```python
from build123d import *

# Parameters (mm, degrees)
ESQUISSE1_R             = 37
ESQUISSE1_R_2           = 1.5
ESQUISSE1_W             = 25
ESQUISSE1_H             = 3
BOSS_EXTRU_1_DEPTH      = 2
BOSS_EXTRU_2_DEPTH      = 15
ESQUISSE3_W             = 1.5
ESQUISSE3_H             = 28.4
ESQUISSE3_W_2           = 1.2
BOSS_EXTRU_3_DEPTH      = 2
ESQUISSE5_W             = 1.5
ESQUISSE5_H             = 24.4
ESQUISSE5_W_2           = 1.2
BOSS_EXTRU_4_DEPTH      = 2
ESQUISSE10_R            = 2
ENL_V_MAT_EXTRU_3_DEPTH = 49
ENL_V_START             = -2
ESQUISSE11_R            = 37
ENL_V_MAT_EXTRU_4_DEPTH = 2
SKETCH4_R               = 3.5
CUT_EXTRUDE2_DEPTH      = 3


with BuildPart() as part:
    # Esquisse1 → Boss.-Extru.1 (new body)
    with BuildSketch(Plane.XY):
        Circle(ESQUISSE1_R)
        with Locations((0, 30)):
            Circle(ESQUISSE1_R_2, mode=Mode.SUBTRACT)
        with Locations((-25.416453209, -15.9375)):
            Circle(ESQUISSE1_R_2, mode=Mode.SUBTRACT)
        with Locations((0, -27)):
            Circle(ESQUISSE1_R_2, mode=Mode.SUBTRACT)
        with Locations((25.416453209, -15.9375)):
            Circle(ESQUISSE1_R_2, mode=Mode.SUBTRACT)
        with Locations((0, -15.5)):
            Rectangle(ESQUISSE1_W, ESQUISSE1_H, mode=Mode.SUBTRACT)
    extrude(amount=BOSS_EXTRU_1_DEPTH)

    # Esquisse2 → Boss.-Extru.2 (add)
    with BuildSketch(Plane(origin=(0, 0, 0), x_dir=(-1, 0, 0), z_dir=(0, 0, -1))):
        Polygon((-22.55, 14.9), (-12.55, 14.9), (-12.55, -9.5), (12.55, -9.5), (12.55, 14.9), (22.55, 14.9), (22.55, -13.5), (-22.55, -13.5), align=None)
    extrude(amount=BOSS_EXTRU_2_DEPTH)

    # Esquisse3 → Boss.-Extru.3 (add)
    with BuildSketch(Plane(origin=(-12.55, 0, 0), x_dir=(0, 0, -1), z_dir=(1, 0, 0))):
        with Locations((9.375, 0.7)):
            Rectangle(ESQUISSE3_W, ESQUISSE3_H)
        with Locations((6.825, 0.7)):
            Rectangle(ESQUISSE3_W_2, ESQUISSE3_H)
    extrude(amount=BOSS_EXTRU_3_DEPTH)

    # Esquisse5 → Boss.-Extru.4 (add)
    with BuildSketch(Plane.ZY.offset(-12.55)):
        with Locations((-9.375, 2.7)):
            Rectangle(ESQUISSE5_W, ESQUISSE5_H)
        with Locations((-6.825, 2.7)):
            Rectangle(ESQUISSE5_W_2, ESQUISSE5_H)
    extrude(amount=BOSS_EXTRU_4_DEPTH)

    # Esquisse10 → Enlèv. mat.-Extru.3 (cut)
    with BuildSketch(Plane.XY.offset(2)):
        with Locations((-17.55, 8.9)):
            Circle(ESQUISSE10_R)
        with Locations((-17.55, -8.5)):
            Circle(ESQUISSE10_R)
        with Locations((17.55, -8.5)):
            Circle(ESQUISSE10_R)
        with Locations((17.55, 8.9)):
            Circle(ESQUISSE10_R)
    extrude(amount=-ENL_V_MAT_EXTRU_3_DEPTH, mode=Mode.SUBTRACT)

    # Esquisse11 → Enlèv. mat.-Extru.4 (cut)
    with BuildSketch(Plane.XY.offset(2).offset(ENL_V_START)):
        Circle(ESQUISSE11_R)
    extrude(amount=ENL_V_MAT_EXTRU_4_DEPTH, mode=Mode.SUBTRACT)

    # Sketch4 → Cut-Extrude2 (cut)
    with BuildSketch(Plane(origin=(0, 0, -15), x_dir=(-1, 0, 0), z_dir=(0, 0, -1))):
        with Locations((-17.55, -8.5)):
            Circle(SKETCH4_R)
        with Locations((-17.55, 8.9)):
            Circle(SKETCH4_R)
        with Locations((17.55, 8.9)):
            Circle(SKETCH4_R)
        with Locations((17.55, -8.5)):
            Circle(SKETCH4_R)
    extrude(amount=-CUT_EXTRUDE2_DEPTH, mode=Mode.SUBTRACT)


solid = part.part
```
Could you check a few things on this model? Use its own coordinates, in mm. A direction names the side the tool comes from. Give positions to 0.01 mm unless a question says otherwise; leave off trailing zeros. Order: outer loops, then holes, each group sorted by start corner. A loop starts at its lowest first (then second) coordinate and runs counter-clockwise, first axis right, second up.
Q1. Suppose I cut it at B-B, the plane y = 13. Write out the boundary of the cut face in (x, z) (3 decimals), and give its area (3 significant figures).
Q2. If I drill on line 1 along Y through (x, z) = (-17.55, -2.75); line 2 along Y through (x, z) = (17.55, -13.6); line 3 along X through (y, z) = (-2, -11.5), over which ranges is the centre line in solid material (lowest first)?
Q3. Suppose I cut it at D-D, the plane x = -8.5. Write out the boundary of the cut face in (y, z).
Q4. For faces 1 (the flat face through (10.55, 3, -9)), 2 (the flat face through (-12, 3, -10.125)), 3 (the flat face through (12, 3, -8.625)), 4 (the flat face through (12.55, 3, -3)), 5 (the cylindrical face through (-19.165, -11.605, -13.521)), which set-ups out of +Z, -Z, +X, -X, +Y, -Y let a thin tool reach every point of the face, with its end or its side?
Q5. I'm going to push flat-ended pins straight in: P1, Ø5.5, axis at x = -17.55, y = 8.9, coming from the +Z side; P2, Ø3.5, axis at x = -19, y = -8.5, coming from the -Z side; P3, Ø0.6, axis at x = 11.5, y = 7.5, coming from the +Z side (3 decimals); P4, Ø1.6, axis at x = -11.5, y = 4.5, coming from the -Z side (3 decimals). Where does each tip first touch, or does it pass through?
Q6. We'd pull the mould along X, two halves only. Please class faces 6 (the flat face through (12.55, 3, -13)), 7 (the flat face through (-18, 14.9, -7)): +X half, -X half, draft (parallel to the pull), parting line (faces both ways), or undercut.
Q7. Suppose I cut it at A-A, the plane x = 17.55. Write out the boundary of the cut face in (y, z).
Q8. Suppose I cut it at C-C, the plane z = -4. Write out the boundary of the cut face in (x, y), and give its area (3 significant figures).
Solution:
1. outline: (-22.55, -15) - (-12.55, -15) - (-12.55, -10.125) - (-10.55, -10.125) - (-10.55, -8.625) - (-12.55, -8.625) - (-12.55, -7.425) - (-10.55, -7.425) - (-10.55, -6.225) - (-12.55, -6.225) - (-12.55, 0) - (-22.55, 0) - close; (10.55, -10.125) - (12.55, -10.125) - (12.55, -15) - (22.55, -15) - (22.55, 0) - (12.55, 0) - (12.55, -6.225) - (10.55, -6.225) - (10.55, -7.425) - (12.55, -7.425) - (12.55, -8.625) - (10.55, -8.625) - close
1. area: 311 mm2
2. line 1: y = -13.5 to -10.5, -6.5 to 6.9, 10.9 to 14.9
2. line 2: y = -13.5 to -12, -5 to 5.4, 12.4 to 14.9
2. line 3: x = -22.55 to -12.55, 12.55 to 22.55
3. outline: (-13.5, -15) - (-9.5, -15) - (-9.5, 0) - (-13.5, 0) - close
4. face 1: +Z, -Z, +Y
4. face 2: -Z, +Y
4. face 3: +Y
4. face 4: +Z, +Y
4. face 5: -Z
5. P1: stops at z = 0
5. P2: stops at z = -12
5. P3: stops at z = -6.225
5. P4: stops at z = -10.125
6. face 6: undercut
6. face 7: draft
7. outline: (-13.5, -15) - (-12, -15) - (-12, -12) - (-10.5, -12) - (-10.5, 0) - (-13.5, 0) - close; (-6.5, -12) - (-5, -12) - (-5, -15) - (5.4, -15) - (5.4, -12) - (6.9, -12) - (6.9, 0) - (-6.5, 0) - close; (10.9, -12) - (12.4, -12) - (12.4, -15) - (14.9, -15) - (14.9, 0) - (10.9, 0) - close
8. outline: (-22.55, -13.5) - (22.55, -13.5) - (22.55, 14.9) - (12.55, 14.9) - (12.55, -9.5) - (-12.55, -9.5) - (-12.55, 14.9) - (-22.55, 14.9) - close; hole circle Ø4 at (-17.55, -8.5); hole circle Ø4 at (-17.55, 8.9); hole circle Ø4 at (17.55, -8.5); hole circle Ø4 at (17.55, 8.9)
8. area: 618 mm2
